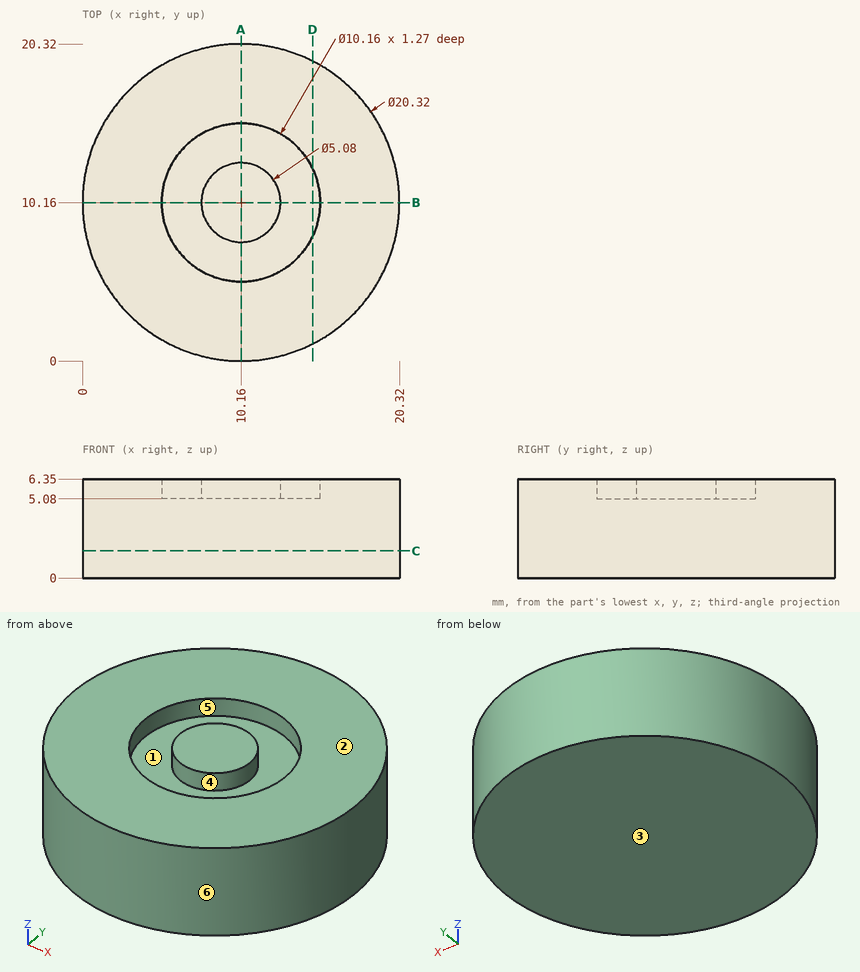
Design review of the part shown in the three views and the two pictorial views. Dimensions are in mm from the part's minimum x, y and z. A direction names the side the tool comes from. Give positions to 0.01 mm unless a question says otherwise; leave off trailing zeros. Write each loop counter-clockwise with the first axis right and the second up, starting at its lowest first coordinate (ties: lowest second). Pieces come first, ordered by that corner, then holes. Notation, with made-up numbers: M -19.75,-31 L -9.75,-31 A25 ccw -9.75,-2 Z; hole C 87.25,43.25 d11. An arc over 180 degrees is marked long. One line per question, with ' | ' between items. Start each with the question number.
Item 1: We need section C-C on z = 1.75. Write out the cut boundary in (x, y), plus the area to 3 significant figures.
Item 2: Wall thickness on line 1 (Y direction, x = 10.16, z = 5.65); line 2 (Z direction, x = 13.75, y = 9.75); line 3 (X direction, y = 10.5, z = 1.5): over which ranges is each line inside the solid? List them lowest first. Write a range as from..to.
Item 3: For the marked faces 1 and 2, list the 3-axis set-ups (+Z, -Z, +X, -X, +Y, -Y) from which the entire face can be reached by the end or side of a thin tool; tool diameter is ignored.
Item 4: We need section A-A on x = 10.16. Write out the cut boundary in (y, z).
Item 5: For pin 1 (1 mm diameter, centred on y = 16, z = 2, fed in from +X); pin 2 (1.5 mm diameter, centred on x = 2.5, z = 5, fed in from -Y), all flat-tipped, find the tip position at first contact; note any pin that passes through.
Item 6: Draft analysis for pull direction X (two halves, no side actions). For the marked faces 3, 4, 5 and 6, state which applies: released by +X, released by -X, zero draft, split by the parting line, or undercut.
Item 7: We need section D-D on x = 14.75. Write out the cut boundary in (y, z), plus the area to 3 significant figures.
Results found:
1) outline: C 10.16,10.16 d20.32 | area: 324 mm2
2) line 1: y = 0..5.08, 7.62..12.7, 15.24..20.32 | line 2: z = 0..5.08 | line 3: x = 0.01..20.31
3) face 1: +Z | face 2: +Z, +X, -X, +Y, -Y
4) outline: M 0,0 L 20.32,0 L 20.32,6.35 L 15.24,6.35 L 15.24,5.08 L 12.7,5.08 L 12.7,6.35 L 7.62,6.35 L 7.62,5.08 L 5.08,5.08 L 5.08,6.35 L 0,6.35 Z
5) pin 1: stops at x = 18.8 | pin 2: stops at y = 2.71
6) face 3: zero draft | face 4: undercut | face 5: undercut | face 6: split by the parting line
7) outline: M 1.1,0 L 19.22,0 L 19.22,6.35 L 12.34,6.35 L 12.34,5.08 L 7.98,5.08 L 7.98,6.35 L 1.1,6.35 Z | area: 110 mm2
